Geometry check sheet. Reference: the model listing, model coordinates, mm. A direction names the side the tool comes from. Give positions to 0.01 mm unless a question says otherwise; leave off trailing zeros. Order: outer loops, then holes, each group sorted by start corner. A loop starts at its lowest first (then second) coordinate and runs counter-clockwise, first axis right, second up. Notation, with made-up numbers: M 11,-25 L 61,-25 A25 ccw 61,5 Z; hole C 15,51 d8. An arc over 180 degrees is marked long. Answer as CSV lines item,"result". Start each with the question number.
```python
from build123d import *

# Parameters (mm, degrees)
F1_DEPTH = 50
F2_R     = 7.5
F3_DEPTH = 50.001
F5_W     = 50
F5_H     = 15
F6_DEPTH = 15


with BuildPart() as f1:
    # F0 (on Front) → F1 (new body)
    with BuildSketch(Plane.XZ):
        Polygon((0, 45), (0, 0), (50, 0), (50, 25), (30, 45), align=None)
    extrude(amount=F1_DEPTH)

    # F2 (on face) → F3 (cut, through all)
    with BuildSketch(Plane.XZ.offset(50)):
        with Locations((20, 20)):
            Circle(F2_R)
    extrude(amount=-F3_DEPTH, mode=Mode.SUBTRACT)

    # F5 (on face) → F6 (cut, through all)
    with BuildSketch(Plane.XY.offset(45)):
        with Locations((25, -32.5)):
            Rectangle(F5_W, F5_H)
    extrude(amount=-F6_DEPTH, mode=Mode.SUBTRACT)


solid = f1.part
```
Item 1: Section check A-A on z = 20. Record the boundary of the cut face in (x, y), then the cut area to 3 significant figures.
Item 2: Access from +Z, -Z, +X, -X, +Y, -Y to the whole of each face (thin tool, end or side, straight path). Record for faces 4 (the face through (17, -25, 38)), 5 (the face through (25, -50, 28)).
Item 3: Section check C-C on y = -26. Record the boundary of the cut face in (x, z).
Item 4: Section check D-D on z = 35. Record the boundary of the cut face in (x, y), then the cut area to 3 significant figures.
Item 5: Depth check by flat-ended pin: pin 1 Ø7.5 at (x, y) = (23, -33) entering from +Z; pin 2 Ø2 at (y, z) = (-11, 30.5) entering from +X. Enter the tip coordinate at first touch or a pass-through.
Item 6: Draft check along Z on faces 1 (the face through (0, -25, 23)), 2 (the face through (22, -32, 30)), 3 (the face through (14.5, -25.4, 25.1)). Enter one of: pulls with the +Z half, pulls with the -Z half, needs draft (parallel to the pull), parting line crosses it, or undercut.
Item 7: Scan lines: line 1 along Y through (x, z) = (21, 40.5); line 2 along Z through (x, y) = (20, -16); line 3 along Z through (x, y) = (20, -33.5). Record each from-to range of solid material in increasing order.
Item 8: Section check B-B on x = 20. Record the boundary of the cut face in (y, z).
Numbers:
1,outline,"M 0,-50 L 12.5,-50 L 12.5,0 L 0,0 Z; M 27.5,-50 L 50,-50 L 50,0 L 27.5,0 Z"
1,area,"1,750 mm2"
2,face 4,"+Z, +X, -X"
2,face 5,"+Z, -Z, +X, -X, -Y"
3,outline,"M 0,0 L 50,0 L 50,25 L 45,30 L 0,30 Z; hole C 20,20 d15"
4,outline,"M 0,-50 L 40,-50 L 40,-40 L 0,-40 Z; M 0,-25 L 40,-25 L 40,0 L 0,0 Z"
4,area,"1,400 mm2"
5,pin 1,"z = 30"
5,pin 2,"x = 45.5"
6,face 1,"needs draft"
6,face 2,"pulls with the +Z half"
6,face 3,"undercut"
7,line 1,"-50 to -40, -25 to 0"
7,line 2,"0 to 12.5, 27.5 to 45"
7,line 3,"0 to 12.5, 27.5 to 30"
8,outline,"M -50,0 L 0,0 L 0,12.5 L -50,12.5 Z; M -50,27.5 L 0,27.5 L 0,45 L -25,45 L -25,30 L -40,30 L -40,45 L -50,45 Z"
